```python
from build123d import *

# Parameters (mm, degrees)
EXTRUDE1_DEPTH = 77.96
EXTRUDE2_DEPTH = 56.175


with BuildPart() as part:
    # Sketch3 → Extrude1 (new body)
    with BuildSketch(Plane(origin=(0, 0, 0), x_dir=(1, 0, 0), z_dir=(0, 1, 0))):
        Polygon((0, 54), (-31.176914536, 36), (-31.176914536, 0), (0, -18), (31.176914536, 0), (31.176914536, 36), align=None)
    extrude(amount=EXTRUDE1_DEPTH)

    # Sketch2 → Extrude2 (add, symmetric)
    with BuildSketch(Plane(origin=(0, 0, 0), x_dir=(0, 0, -1), z_dir=(1, 0, 0))):
        Polygon((0, 10), (42.426406871, 52.426406871), (-15.529142706, 67.955549577), align=None)
    extrude(amount=EXTRUDE2_DEPTH, both=True)


solid = part.part
```
The listing builds one solid part. Answer for the finished solid, in the listing's coordinates (mm). A direction names the side the tool comes from. Give positions to 0.01 mm unless a question says otherwise; leave off trailing zeros. Order: outer loops, then holes, each group sorted by start corner. A loop starts at its lowest first (then second) coordinate and runs counter-clockwise, first axis right, second up. Notation, with made-up numbers: (80, -11) -> (113, -11) arc R18 cw to (113, 15) -> close; hole circle Ø2 at (26.5, -27.5). An arc over 180 degrees is marked (long way). Answer as a JSON object with one key per item and string values. Group by question number.
Item 1: Flat-ended cylindrical pins translate along their axes: pin 1 (19 mm diameter, centred on y = 71.5, z = -18.5, fed in from +X); pin 2 (12 mm diameter, centred on x = -26, y = 11.5, fed in from -Z); pin 3 (8 mm diameter, centred on x = 17, y = 33, fed in from -Z). Find the tip coordinate at first contact, or state that the pin passes through.
Item 2: A tool of negligible diameter and unlimited length cuts with its end or side. For faces 1 (the flat face through (-41.396, 60.082, -13.854)), 2 (the flat face through (-31.177, 69, -18)), 3 (the flat face through (-35.63, 39.383, 7.873)), 4 (the flat face through (31.177, 69, -18)), from which of +Z, -Z, +X, -X, +Y, -Y can it reach the whole face along a straight path? Write none if from no direction.
Item 3: The part is cut by section C-C on x = 11. Write down the section's boundary in (y, z).
Item 4: Determine the mould class of faces 5 (the flat face through (36.357, 39.383, 7.873)), 6 (the flat face through (42, 31, -21)), 7 (the flat face through (-56.175, 46, -7)) for opening direction Z: pulls with the +Z half, pulls with the -Z half, needs draft (parallel to the pull), parting line crosses it, or undercut.
Item 5: Consider L1, parallel to X at y = 13, z = -32.5; L2, parallel to Z at x = -21, y = 49.5; L3, parallel to Y at x = -31.5, z = -12.5. Determine where each line is inside the solid, lowest interval first. Write a range as from..to.
Item 6: The part is cut by section D-D on y = 15.5. Write down the section's boundary in (x, z) (3 decimals), and give its area (3 significant figures).
Item 7: The part is cut by section A-A on y = 6.5. Write down the section's boundary in (x, z), and give its area (3 significant figures).
Item 8: The part is cut by section B-B on z = -26.5. Write down the section's boundary in (x, y) (3 decimals), and give its area (3 significant figures).
Result set:
{
 "1": {"pin 1": "x = 31.18", "pin 2": "z = -42.45", "pin 3": "z = -46.49"},
 "2": {"face 1": "-X, +Y", "face 2": "-Z, -X, +Y", "face 3": "+Z, -X, -Y", "face 4": "-Z, +X, +Y"},
 "3": {"outline": "(0, -47.65) -> (77.96, -47.65) -> (77.96, 11.65) -> (66.92, 11.65) -> (67.96, 15.53) -> (53.48, 11.65) -> (0, 11.65) -> close"},
 "4": {"face 5": "pulls with the +Z half", "face 6": "pulls with the -Z half", "face 7": "needs draft"},
 "5": {"L1": "-31.18..31.18", "L2": "-41.88..10.58", "L3": "22.5..60.45"},
 "6": {"outline": "(-56.175, -5.5) -> (-31.177, -5.5) -> (-31.177, -36) -> (0, -54) -> (31.177, -36) -> (31.177, -5.5) -> (56.175, -5.5) -> (56.175, 1.474) -> (28.624, 1.474) -> (0, 18) -> (-28.624, 1.474) -> (-56.175, 1.474) -> close", "area": "3,720 mm²"},
 "7": {"outline": "(-31.18, -36) -> (0, -54) -> (31.18, -36) -> (31.18, 0) -> (0, 18) -> (-31.18, 0) -> close", "area": "3,370 mm²"},
 "8": {"outline": "(-56.175, 36.5) -> (-31.177, 36.5) -> (-31.177, 0) -> (31.177, 0) -> (31.177, 36.5) -> (56.175, 36.5) -> (56.175, 56.694) -> (31.177, 56.694) -> (31.177, 77.96) -> (-31.177, 77.96) -> (-31.177, 56.694) -> (-56.175, 56.694) -> close", "area": "5,870 mm²"}
}
